from build123d import *

# Parameters (mm, degrees)
SKETCH_1_R      = 14
EXTRUDE_1_DEPTH = 19.3
SKETCH_3_R      = 2
EXTRUDE_2_DEPTH = 1
SKETCH_4_R      = 4.5
EXTRUDE_3_DEPTH = 1.5
SKETCH_6_W      = 14.6
SKETCH_6_H      = 5.55387092
EXTRUDE_4_DEPTH = 19.3


with BuildPart() as part:
    # 草图1 → 凸台-拉伸1 (new body)
    with BuildSketch(Plane.XY):
        with Locations((-50.023496645, 38.50258845)):
            Circle(SKETCH_1_R)
    extrude(amount=EXTRUDE_1_DEPTH)

    # 草图3 → 凸台-拉伸2 (add)
    with BuildSketch(Plane.XY.offset(19.3)):
        with BuildLine():
            Line((-63.578938357, 42.00258845), (-67.523496645, 42.00258845))
            ThreePointArc((-67.523496645, 42.00258845), (-71.023496645, 38.50258845), (-67.523496645, 35.00258845))
            Line((-67.523496645, 35.00258845), (-63.578938357, 35.00258845))
            ThreePointArc((-63.578938357, 35.00258845), (-64.023496645, 38.50258845), (-63.578938357, 42.00258845))
        make_face()
        with Locations((-67.523496645, 38.50258845)):
            Circle(SKETCH_3_R, mode=Mode.SUBTRACT)
        with BuildLine():
            Line((-32.523496645, 42.00258845), (-36.468054934, 42.00258845))
            ThreePointArc((-36.468054934, 42.00258845), (-36.135080898, 40.266648545), (-36.023496645, 38.50258845))
            ThreePointArc((-36.023496645, 38.50258845), (-36.135080898, 36.738528355), (-36.468054934, 35.00258845))
            Line((-36.468054934, 35.00258845), (-32.523496645, 35.00258845))
            ThreePointArc((-32.523496645, 35.00258845), (-29.023496645, 38.50258845), (-32.523496645, 42.00258845))
        make_face()
        with Locations((-32.523496645, 38.50258845)):
            Circle(SKETCH_3_R, mode=Mode.SUBTRACT)
        with BuildLine():
            ThreePointArc((-42.723496645, 26.55645937), (-50.023496645, 24.50258845), (-57.323496645, 26.55645937))
            Line((-57.323496645, 26.55645937), (-57.323496645, 21.00258845))
            Line((-57.323496645, 21.00258845), (-42.723496645, 21.00258845))
            Line((-42.723496645, 21.00258845), (-42.723496645, 26.55645937))
        make_face()
    extrude(amount=-EXTRUDE_2_DEPTH)

    # 草图4 → 凸台-拉伸3 (add)
    with BuildSketch(Plane.XY.offset(19.3)):
        with Locations((-50.023496645, 46.50258845)):
            Circle(SKETCH_4_R)
    extrude(amount=EXTRUDE_3_DEPTH)

    # 草图6 → 凸台-拉伸4 (add)
    with BuildSketch(Plane.XY.offset(19.3)):
        with Locations((-50.023496645, 23.77952391)):
            Rectangle(SKETCH_6_W, SKETCH_6_H)
    extrude(amount=-EXTRUDE_4_DEPTH)


solid = part.part
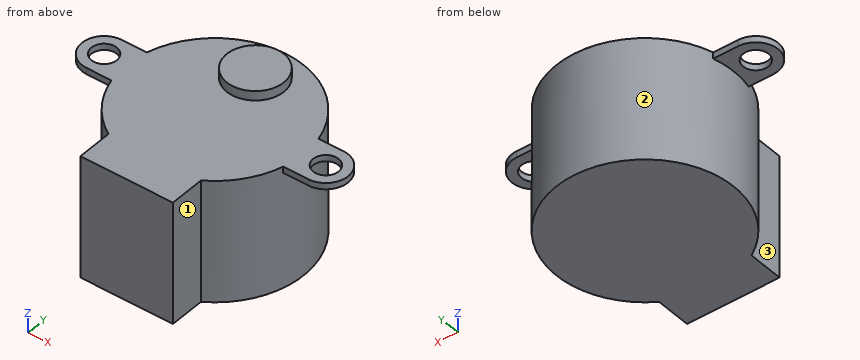
For this review, take the finished solid that the model builds, in its own axes (mm). Face numbers are marked on the shaded views. A direction names the side the tool comes from. Give positions to 0.01 mm unless a question says otherwise; leave off trailing zeros. Loops run counter-clockwise (first coordinate to the right, second up) from the corner with the lowest first, then second, coordinate; pieces in that order, holes last. Notation, with made-up numbers: M 77,37.25 L 132,37.25 A24 ccw 132,67.25 Z; hole C -23.75,-12.5 d5. An arc over 180 degrees is marked long. Answer as a JSON object with one key per item and string values. Group by question number.
Q1. Insertion check: P1, Ø2, axis at y = 46, z = 14.5, coming from the -X side; P2, Ø2, axis at x = -51, z = 5, coming from the +Y side; P3, Ø0.8, axis at x = -33.5, z = 18.5, coming from the +Y side; P4, Ø10, axis at y = 26.5, z = 5, coming from the -X side. Each pin has a flat end and moves straight along its axis. Give the tip position at first contact, or say it passes through.
Q2. Add section A-A on y = 48.5. Give the boundary of the cut face in (x, z), and give its area (3 significant figures).
Q3. Tool access review of the marked faces 1, 2 and 3: name each direction out of +Z, -Z, +X, -X, +Y, -Y from which nothing blocks a thin tool from reaching the whole face with its end or side.
Q4. Add section B-B on z = 13.5. Give the boundary of the cut face in (x, y).
Q5. Add section D-D on x = -50.5. Give the boundary of the cut face in (y, z).
Q6. For probe 1 along Z at (x, y) = (-56, 28.5); probe 2 along X at (y, z) = (35, 14.5); probe 3 along Y at (x, z) = (-37.5, 18.25), list the stretches that pass through material, from the lowest coordinate up. Write a range as [from, to].
Q7. Add section C-C on x = -35. Give the boundary of the cut face in (y, z).
Checked values:
{
 "1": {"P1": "x = -62.42", "P2": "y = 52.5", "P3": "y = 42", "P4": "x = -62.15"},
 "2": {"outline": "M -59.82,0 L -40.22,0 L -40.22,19.3 L -45.99,19.3 L -45.99,20.8 L -54.06,20.8 L -54.06,19.3 L -59.82,19.3 Z", "area": "390 mm²"},
 "3": {"face 1": "+Z, -Z, +X, -Y", "face 2": "-Z", "face 3": "+Z, -Z, -X, -Y"},
 "4": {"outline": "M -57.32,21 L -42.72,21 L -42.72,26.56 A14 ccw long -57.32,26.56 Z"},
 "5": {"outline": "M 21,0 L 52.49,0 L 52.49,19.3 L 50.98,19.3 L 50.98,20.8 L 42.03,20.8 L 42.03,19.3 L 21,19.3 Z"},
 "6": {"probe 1": "[0, 19.3]", "probe 2": "[-63.58, -36.47]", "probe 3": "[32.24, 44.76]"},
 "7": {"outline": "M 35,18.3 L 42,18.3 L 42,19.3 L 35,19.3 Z"}
}
